```python
from build123d import *

# Parameters (mm, degrees)
F4_DEPTH = 10
F3_W     = 0.9957388944
F3_H     = 7.3437828345
F5_DEPTH = 10
F6_DEPTH = 10


with BuildPart() as f1:
    # F0 (on Top) → F1 (revolve)
    with BuildSketch(Plane.XY):
        with BuildLine():
            Line((-25, 0), (25, 0))
            ThreePointArc((25, 0), (0, 25), (-25, 0))
        make_face()
    revolve(axis=Axis((0, 0, 0), (-1, 0, 0)))

    # F3 (on offset) → F4 (cut)
    with BuildSketch(Plane.XZ.offset(25)):
        with BuildLine():
            Line((-2.1299138496, -3.89204987), (-1.0190895553, -3.89204987))
            Line((-1.0190895553, -3.89204987), (1.0858057291, 1.7471347231))
            Line((1.0858057291, 1.7471347231), (0.0900668347, 1.7471347231))
            Line((0.0900668347, 1.7471347231), (-1.1908837029, -1.9322622637))
            Line((-1.1908837029, -1.9322622637), (-1.3943680331, -2.5477189673))
            Line((-1.3943680331, -2.5477189673), (-1.5778375111, -3.1565040535))
            add(Edge.make_bspline(
                [(-1.9364369455, -1.9222548377), (-1.8697207716, -2.1307428809), (-1.5778375111, -3.1565040535)],
                knots=[0, 0, 0, 1, 1, 1], degree=2))
            Line((-1.9364369455, -1.9222548377), (-3.1773577787, 1.7471347231))
            Line((-3.1773577787, 1.7471347231), (-4.1781003862, 1.7471347231))
            Line((-4.1781003862, 1.7471347231), (-2.1299138496, -3.89204987))
        make_face()
    extrude(amount=-F4_DEPTH, mode=Mode.SUBTRACT)

    # F3 (on offset) → F5 (cut)
    with BuildSketch(Plane.XZ.offset(25)):
        with Locations((-5.6967272931, -0.2201584528)):
            Rectangle(F3_W, F3_H)
    extrude(amount=-F5_DEPTH, mode=Mode.SUBTRACT)

    # F3 (on offset) → F6 (cut)
    with BuildSketch(Plane.XZ.offset(25)):
        with BuildLine():
            add(Edge.make_bspline(
                [(2.1182385192, -6.1070268413), (1.7329526153, -6.1070268413), (1.471091633, -6.0503180935)],
                knots=[0, 0, 0, 1, 1, 1], degree=2))
            add(Edge.make_bspline(
                [(2.9496888355, -5.8910332285), (2.5819159273, -6.1070268413), (2.1182385192, -6.1070268413)],
                knots=[0, 0, 0, 1, 1, 1], degree=2))
            add(Edge.make_bspline(
                [(3.6193524304, -5.2347128684), (3.3174617438, -5.6750396157), (2.9496888355, -5.8910332285)],
                knots=[0, 0, 0, 1, 1, 1], degree=2))
            add(Edge.make_bspline(
                [(4.2715030296, -3.89204987), (3.921243117, -4.7943861211), (3.6193524304, -5.2347128684)],
                knots=[0, 0, 0, 1, 1, 1], degree=2))
            Line((4.2715030296, -3.89204987), (6.4397786791, 1.7471347231))
            Line((6.4397786791, 1.7471347231), (5.4490434977, 1.7471347231))
            Line((5.4490434977, 1.7471347231), (4.2131263775, -1.8438633334))
            Line((4.2131263775, -1.8438633334), (3.8478553258, -2.8696245061))
            add(Edge.make_bspline(
                [(3.6351975217, -2.2241455242), (3.8328441866, -2.8029083322), (3.8478553258, -2.8696245061)],
                knots=[0, 0, 0, 1, 1, 1], degree=2))
            add(Edge.make_bspline(
                [(3.4008569611, -1.5436405512), (3.4375508567, -1.6453827163), (3.6351975217, -2.2241455242)],
                knots=[0, 0, 0, 1, 1, 1], degree=2))
            add(Edge.make_bspline(
                [(3.3374765959, -1.3685105949), (3.3641630655, -1.4418983861), (3.4008569611, -1.5436405512)],
                knots=[0, 0, 0, 1, 1, 1], degree=2))
            Line((3.3374765959, -1.3685105949), (2.1499287017, 1.7471347231))
            Line((2.1499287017, 1.7471347231), (1.1491860943, 1.7471347231))
            Line((1.1491860943, 1.7471347231), (3.3841779176, -3.8653634005))
            Line((3.3841779176, -3.8653634005), (3.2957789873, -4.0905304872))
            add(Edge.make_bspline(
                [(1.9097504759, -5.3781526422), (2.7854002575, -5.3781526422), (3.2957789873, -4.0905304872)],
                knots=[0, 0, 0, 1, 1, 1], degree=2))
            add(Edge.make_bspline(
                [(1.471091633, -5.3464624596), (1.6695722501, -5.3781526422), (1.9097504759, -5.3781526422)],
                knots=[0, 0, 0, 1, 1, 1], degree=2))
            Line((1.471091633, -5.3464624596), (1.471091633, -6.0503180935))
        make_face()
    extrude(amount=-F6_DEPTH, mode=Mode.SUBTRACT)


solid = f1.part
```
Check sheet for the modelled part. Datum: model origin and axes. Units: mm. Coordinates: 2 decimals unless noted, no trailing zeros. Order: outer loops, then holes, each group sorted by start corner. A loop starts at its lowest first (then second) coordinate and runs counter-clockwise, first axis right, second up. Notation, with made-up numbers: M 44.5,24 L 93.5,24 A18 cw 93.5,32 Z; hole C 59,29 d6. An arc over 180 degrees is marked long. Write each question's results on one line, items separated by ' | '. Start each with the question number.
1. Material ranges on probe 1 along Z at (x, y) = (18.5, -7); probe 2 along Y at (x, z) = (10, 20); probe 3 along Z at (x, y) = (-10.5, 4), recorded low to high.
2. Mould release check, pull along Z, two halves, no side actions. Record for faces 1 (the face through (-5.199, -20, 0)), 2 (the face through (4.84, -19.86, -0.02)): +Z half, -Z half, draft (parallel to the pull), parting line (faces both ways), or undercut.
3. Cross-section at B-B on y = -20. State how many separate pieces and enclosed holes the cut face has, and give its area (3 significant figures).
4. Cross-section at A-A on z = 15. Record the cut outline in (x, y).
5. Cross-section at C-C on x = 18. Record the cut outline in (y, z).
6. Go/stop test with flat-tipped pins: P1, Ø6, axis at y = -18, z = 0, coming from the +X side; P2, Ø2, axis at x = -2, z = -12, coming from the -Y side; P3, Ø10, axis at x = -16.5, z = 14, coming from the +Y side. Record where each tip stops, or that it passes through.
Checks:
1) probe 1: z = -15.29 to 15.29 | probe 2: y = -11.18 to 11.18 | probe 3: z = -22.33 to 22.33
2) face 1: undercut | face 2: undercut
3) separate pieces: 1 | enclosed holes: 3 | area: 677 mm²
4) outline: C 0,0 d40
5) outline: C 0,0 d34.7
6) P1: stops at x = 20 | P2: stops at y = -22.37 | P3: stops at y = 18.66
